```python
from build123d import *

# Parameters (mm, degrees)
F0_W     = 70
F0_H     = 55
F0_R     = 1.55
F1_DEPTH = 8
F2_R     = 4
F3_DEPTH = 5
F4_W     = 60
F4_H     = 1.6
F5_DEPTH = 5
F6_W     = 60
F6_H     = 2.5
F7_DEPTH = 3


with BuildPart() as f1:
    # F0 (on Top) → F1 (new body)
    with BuildSketch(Plane.XY):
        Rectangle(F0_W, F0_H)
        with Locations((-30, -12.5)):
            Circle(F0_R, mode=Mode.SUBTRACT)
        with Locations((-15, -12.5)):
            Circle(F0_R, mode=Mode.SUBTRACT)
        with Locations((0, -12.5)):
            Circle(F0_R, mode=Mode.SUBTRACT)
        with Locations((15, -12.5)):
            Circle(F0_R, mode=Mode.SUBTRACT)
        with Locations((30, -12.5)):
            Circle(F0_R, mode=Mode.SUBTRACT)
        with Locations((-30, 12.5)):
            Circle(F0_R, mode=Mode.SUBTRACT)
        with Locations((-15, 12.5)):
            Circle(F0_R, mode=Mode.SUBTRACT)
        with Locations((0, 12.5)):
            Circle(F0_R, mode=Mode.SUBTRACT)
        with Locations((15, 12.5)):
            Circle(F0_R, mode=Mode.SUBTRACT)
        with Locations((30, 12.5)):
            Circle(F0_R, mode=Mode.SUBTRACT)
    extrude(amount=F1_DEPTH)

    # F2 (on face) → F3 (cut)
    with BuildSketch(Plane.XY.offset(8)):
        with Locations((0, -12.5)):
            Circle(F2_R)
        with Locations((0, 12.5)):
            Circle(F2_R)
        with Locations((15, -12.5)):
            Circle(F2_R)
        with Locations((30, -12.5)):
            Circle(F2_R)
        with Locations((-15, -12.5)):
            Circle(F2_R)
        with Locations((-30, -12.5)):
            Circle(F2_R)
        with Locations((15, 12.5)):
            Circle(F2_R)
        with Locations((30, 12.5)):
            Circle(F2_R)
        with Locations((-15, 12.5)):
            Circle(F2_R)
        with Locations((-30, 12.5)):
            Circle(F2_R)
    extrude(amount=-F3_DEPTH, mode=Mode.SUBTRACT)

    # F4 (on face) → F5 (cut)
    with BuildSketch(Plane.XY.offset(8)):
        with Locations((0, -21.7)):
            Rectangle(F4_W, F4_H)
        with Locations((0, -23.3)):
            Rectangle(F4_W, F4_H)
        with Locations((0, 21.7)):
            Rectangle(F4_W, F4_H)
        with Locations((0, 23.3)):
            Rectangle(F4_W, F4_H)
    extrude(amount=-F5_DEPTH, mode=Mode.SUBTRACT)

    # F6 (on face) → F7 (cut)
    with BuildSketch(Plane(origin=(0, 0, 0), x_dir=(1, 0, 0), z_dir=(0, 0, -1))):
        Polygon((-30, 22.5), (-30, 20), (30, 20), (30, 22.5), (30, 25), (-30, 25), align=None)
        with Locations((0, -21.25)):
            Rectangle(F6_W, F6_H)
        with Locations((0, -23.75)):
            Rectangle(F6_W, F6_H)
    extrude(amount=-F7_DEPTH, mode=Mode.SUBTRACT)


solid = f1.part
```
For this review, take the finished solid that the model builds, in its own axes (mm). A direction names the side the tool comes from. Round coordinates to 2 decimals unless told otherwise and drop trailing zeros. Write each loop counter-clockwise with the first axis right and the second up, starting at its lowest first coordinate (ties: lowest second). Pieces come first, ordered by that corner, then holes. Notation, with made-up numbers: (-3, 16.25) - (37, 16.25) arc R16 ccw to (37, 47.25) - close; hole circle Ø2 at (6.5, -26). An arc over 180 degrees is marked (long way). Write each question's results on one line, items separated by ' | '.
Item 1: For faces 3 (the face through (0, 25, 1)), 4 (the face through (-0.867, -16.405, 5.535)), 5 (the face through (0, -20.9, 6)), list the 3-axis set-ups (+Z, -Z, +X, -X, +Y, -Y) from which the entire face can be reached by the end or side of a thin tool; tool diameter is ignored.
Calculated:
face 3: -Z | face 4: +Z | face 5: +Z, -Z
Item 2: Take a section at B-B on z = 3.75. Count the separate pieces of the cut face and the enclosed holes in it, then the cut area to 3 significant figures.
Calculated:
separate pieces: 1 | enclosed holes: 12 | area: 2,960 mm^2
Item 3: For pin 1 (2.5 mm diameter, centred on x = 29, y = -11.5, fed in from +Z), flat-tipped, find the tip position at first contact; note if it passes through.
Calculated:
pin 1: stops at z = 3
Item 4: Draft analysis for pull direction X (two halves, no side actions). For faces 1 (the face through (0, -27.5, 4)), 2 (the face through (32, 13, 3)), state which applies: pulls with the +X half, pulls with the -X half, needs draft (parallel to the pull), parting line crosses it, or undercut.
Calculated:
face 1: needs draft | face 2: undercut
Item 5: To check wall thickness, follow line 1 along Y through (x, z) = (-13, 1.75); line 2 along Y through (x, z) = (-5.5, 4); line 3 along Y through (x, z) = (0, 6.6). State the ranges of each line that lie inside material, in increasing order. Write a range as from..to.
Calculated:
line 1: y = -27.5..-25, -20..20, 25..27.5 | line 2: y = -27.5..-24.1, -20.9..20.9, 24.1..27.5 | line 3: y = -27.5..-24.1, -20.9..-16.5, -8.5..8.5, 16.5..20.9, 24.1..27.5
Item 6: Take a section at A-A on x = 9. State the section outline as (y, z) points, then the cut area to 3 significant figures.
Calculated:
outline: (-27.5, 0) - (-25, 0) - (-25, 3) - (-24.1, 3) - (-24.1, 8) - (-27.5, 8) - close; (-20.9, 3) - (-20, 3) - (-20, 0) - (20, 0) - (20, 3) - (20.9, 3) - (20.9, 8) - (-20.9, 8) - close; (24.1, 3) - (25, 3) - (25, 0) - (27.5, 0) - (27.5, 8) - (24.1, 8) - close | area: 378 mm^2
